Build history of the part. All positions in model axes, mm. Give positions to 0.01 mm unless a question says otherwise; leave off trailing zeros. Order: outer loops, then holes, each group sorted by start corner. A loop starts at its lowest first (then second) coordinate and runs counter-clockwise, first axis right, second up. Notation, with made-up numbers: (12, -33.5) -> (36, -33.5) arc R31 cw to (36, 2.5) -> close; hole circle Ø9 at (10.5, 57.5). An arc over 180 degrees is marked (long way). One line per question, with ' | ' between items. Start each with the question number.
(1) Pin check, flat tips, straight feed: pin 1 Ø5 at (y, z) = (-10.5, -12) entering from +X; pin 2 Ø5 at (x, z) = (-10, -1.5) entering from +Y; pin 3 Ø8 at (x, y) = (9, 3.5) entering from +Z. Stop position of each tip, or through.
(2) Cut at D-D (y = 0). Give the cut face in (x, z).
(3) Cut at B-B (x = -1). Give the cut face in (y, z).
(4) Cut at C-C (y = 7). Give the cut face in (x, z).
(5) Drill centre lines: L1, parallel to Y at x = 3.75, z = 4.75; L2, parallel to Y at x = -4.25, z = 12; L3, parallel to Z at x = -6, y = 1.75. Where is each one in solid material? Low to high. Write a range as from..to.
(6) Cut at A-A (z = -7.5). Give the cut face in (x, y), then the cut area to 3 significant figures.
from build123d import *

# Parameters (mm, degrees)
F4_T     = -1
F3_R     = 8.042846649
F5_DEPTH = 25.4


with BuildPart() as f1:
    # F0 (on Right) → F1 (revolve)
    with BuildSketch(Plane.YZ):
        with BuildLine():
            ThreePointArc((0, -15), (10.6066017178, -10.6066017178), (15, 0))
            ThreePointArc((15, 0), (10.6066017178, 10.6066017178), (0, 15))
            Line((0, 15), (0, -15))
        make_face()
    revolve(axis=Axis((0, 0, 0), (0, 0, -1)))

    # F4 (hollow: no face is removed)
    offset(amount=F4_T, mode=Mode.SUBTRACT)

    # F3 (on offset) → F5 (cut)
    with BuildSketch(Plane.YZ.offset(12.446)):
        Circle(F3_R)
    extrude(amount=F5_DEPTH, mode=Mode.SUBTRACT)


solid = f1.part
Result set:
1) pin 1: stops at x = 6.65 | pin 2: stops at y = 12.93 | pin 3: stops at z = 13.89
2) outline: (12.45, -8.04) -> (12.45, -6.41) arc R14 cw (long way) to (12.45, 6.41) -> (12.45, 8.04) -> (12.66, 8.04) arc R15 ccw (long way) to (12.66, -8.04) -> close
3) outline: circle Ø29.93 at (0, 0); hole circle Ø27.93 at (0, 0)
4) outline: (12.45, -3.96) -> (12.45, 3.96) -> (12.66, 3.96) arc R13.27 ccw (long way) to (12.66, -3.96) -> close; hole circle Ø24.25 at (0, 0)
5) L1: y = -13.72..-12.62, 12.62..13.72 | L2: y = -7.93..-5.83, 5.83..7.93 | L3: z = -13.64..-12.53, 12.53..13.64
6) outline: (12.45, -2.9) -> (12.45, 2.9) -> (12.66, 2.9) arc R12.99 ccw (long way) to (12.66, -2.9) -> close; hole circle Ø23.64 at (0, 0) | area: 88.6 mm2
